Part model, mm, in its own coordinate system. A direction names the side the tool comes from. Coordinates: 2 decimals unless noted, no trailing zeros. Write each loop counter-clockwise with the first axis right and the second up, starting at its lowest first coordinate (ties: lowest second). Pieces come first, ordered by that corner, then holes. Notation, with made-up numbers: M -3.75,37 L 9.25,37 A16 cw 9.25,47 Z; hole C 80,20 d8. An arc over 180 degrees is marked long. Use a Markdown table: item, result. Add a question column.
Q1. Slice it at A-A on x = 748. Write the cut outline in (y, z).
Q2. Pin check, flat tips, straight feed: pin 1 Ø14.5 at (x, z) = (1130, -23.81) entering from -Y; pin 2 Ø8 at (x, z) = (470.5, -7.5) entering from +Y; pin 3 Ø6 at (x, y) = (-747, -4.5) entering from +Z. Stop position of each tip, or through.
Q3. Slice it at B-B on y = -1.5. Write the cut outline in (x, z), then the cut area to 3 significant figures.
Q4. Wall check: L1, parallel to Z at x = 1130, y = -15.05; L2, parallel to Z at x = 1130, y = -15.15; L3, parallel to Y at x = -475, z = -49.5. Give the ranges that are in metal, low to high. Write a range as from..to.
Q5. Tool access for faces 1 (the flat face through (16, -14.214, -12)), 2 (the flat face through (16, -15.714, -13)): list every direction of +Z, -Z, +X, -X, +Y, -Y with a clear straight run to the whole face (end or side of a thin tool).
from build123d import *

# Parameters (mm, degrees)
EXTRUDE_THIN1_DEPTH = 1150
FILLET1_R           = 1.5
FILLET2_R           = 3
SKETCH2_R           = 4.5
CUT_EXTRUDE1_DEPTH  = 10


with BuildPart() as part:
    # Sketch1 → Extrude-Thin1 (new, symmetric)
    with BuildSketch(Plane(origin=(0, 0, 0), x_dir=(0, 0, -1), z_dir=(1, 0, 0))):
        Polygon((63.80952381, 24.285714286), (63.80952381, -15.714285714), (-36.19047619, -15.714285714), (-36.19047619, -14.214285714), (62.30952381, -14.214285714), (62.30952381, 24.285714286), align=None)
    extrude(amount=EXTRUDE_THIN1_DEPTH, both=True)

    # Fillet1
    fillet1_edges = [part.edges().sort_by_distance(p)[0] for p in [
        (0, -14.214285714, -62.30952381),
    ]]
    fillet(fillet1_edges, radius=FILLET1_R)

    # Fillet2
    fillet2_edges = [part.edges().sort_by_distance(p)[0] for p in [
        (0, -15.714285714, -63.80952381),
    ]]
    fillet(fillet2_edges, radius=FILLET2_R)

    # Sketch2 → Cut-Extrude1 (cut)
    with BuildSketch(Plane(origin=(0, -14.214285714, 0), x_dir=(1, 0, 0), z_dir=(0, 1, 0))):
        with Locations(Location((-1130, 23.80952381, 0), (0, 0, 270))):
            Circle(SKETCH2_R)
    cut_extrude1 = extrude(amount=-CUT_EXTRUDE1_DEPTH, mode=Mode.SUBTRACT)

    # Mirror1: Cut-Extrude1 across plane
    add(cut_extrude1.mirror(Plane(origin=(0, 0, 0), x_dir=(0, 0, 1), z_dir=(1, 0, 0))), mode=Mode.SUBTRACT)


solid = part.part
Recorded:
| question | item | result |
|---|---|---|
| 1 | outline | M -15.71,-60.81 A3 ccw -12.71,-63.81 L 24.29,-63.81 L 24.29,-62.31 L -12.71,-62.31 A1.5 cw -14.21,-60.81 L -14.21,36.19 L -15.71,36.19 Z |
| 2 | pin 1 | y = -15.71 |
| 2 | pin 2 | y = -14.21 |
| 2 | pin 3 | z = -62.31 |
| 3 | outline | M -1150,-63.81 L 1150,-63.81 L 1150,-62.31 L -1150,-62.31 Z |
| 3 | area | 3,450 mm² |
| 4 | L1 | -62.69..-28.31, -19.31..36.19 |
| 4 | L2 | -62.56..-28.31, -19.31..36.19 |
| 4 | L3 | -15.71..-14.21 |
| 5 | face 1 | +Z, +X, -X, +Y |
| 5 | face 2 | +Z, -Z, +X, -X, -Y |
